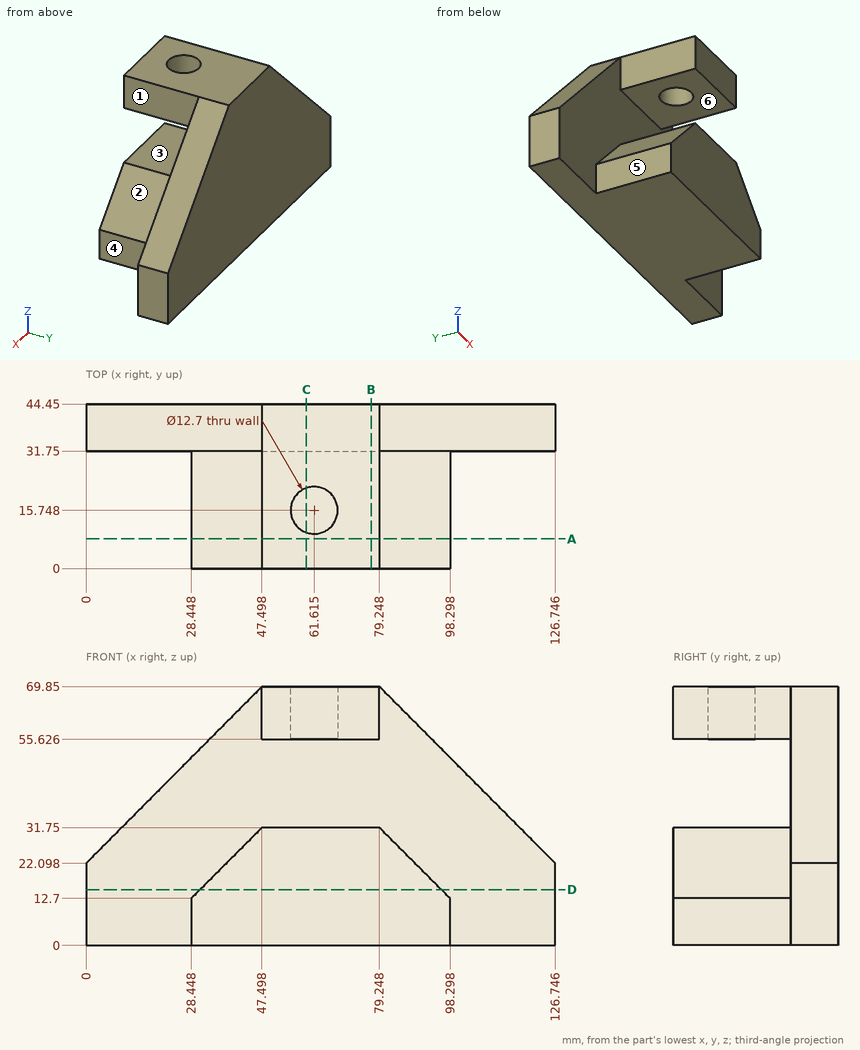
Input: dimensioned drawing with shaded views. Units: mm. Origin: part minimum x, y, z. A direction names the side the tool comes from. Coordinates: 2 decimals unless noted, no trailing zeros. Loops run counter-clockwise (first coordinate to the right, second up) from the corner with the lowest first, then second, coordinate; pieces in that order, holes last. Notation, with made-up numbers: M 32.25,28.5 L 56.25,28.5 A16 ccw 56.25,37.5 Z; hole C 12.25,-22 d4. An arc over 180 degrees is marked long. Use a Markdown table: item, result. Add a question column.
1) Section D-D, the plane z = 15. Return the cut outline in (x, y).
2) Draft query along Z for the marked faces 1, 2 and 3. Return one class per face: +Z half, -Z half, draft (parallel to the pull), parting line (faces both ways), or undercut.
3) Section B-B, the plane x = 77. Return the cut outline in (y, z), plus the area to 3 significant figures.
4) Pin query (flat end, axial travel): P1, Ø12, axis at x = 100.5, y = 8.5, coming from the +Z side; P2, Ø6, axis at y = 15, z = 59, coming from the -X side; P3, Ø7, axis at y = 12.5, z = 62.5, coming from the +X side; P4, Ø1.5, axis at x = 100, y = 5, coming from the -Z side. Return the tip coordinate at first contact, or that it passes through.
5) Line query: L1, parallel to Z at x = 64, y = 31.5; L2, parallel to Y at x = 41, z = 55; L3, parallel to X at y = 29, z = 59.5. Output: solid intervals per line, ascending. Write a range as from..to.
6) Section C-C, the plane x = 59.5. Return the cut outline in (y, z), plus the area to 3 significant figures.
7) Set-up query: the marked faces 4, 5 and 6. Return all of +Z, -Z, +X, -X, +Y, -Y with unobstructed straight access to the full face (end or side cutting, diameter ignored); none if empty.
8) Section A-A, the plane y = 8. Return the cut outline in (x, z).
Answer below:
| question | item | result |
|---|---|---|
| 1 | outline | M 0,31.75 L 30.75,31.75 L 30.75,0 L 96,0 L 96,31.75 L 126.75,31.75 L 126.75,44.45 L 0,44.45 Z |
| 2 | face 1 | draft |
| 2 | face 2 | +Z half |
| 2 | face 3 | undercut |
| 3 | outline | M 0,0 L 44.45,0 L 44.45,69.85 L 0,69.85 L 0,55.63 L 31.75,55.63 L 31.75,31.75 L 0,31.75 Z |
| 3 | area | 2,350 mm2 |
| 4 | P1 | z = 16.5 |
| 4 | P2 | x = 47.5 |
| 4 | P3 | x = 79.25 |
| 4 | P4 | through |
| 5 | L1 | 0..31.75, 55.63..69.85 |
| 5 | L2 | 31.75..44.45 |
| 5 | L3 | 47.5..79.25 |
| 6 | outline | M 0,0 L 44.45,0 L 44.45,69.85 L 21.74,69.85 L 21.74,55.63 L 31.75,55.63 L 31.75,31.75 L 0,31.75 Z; M 0,55.63 L 9.76,55.63 L 9.76,69.85 L 0,69.85 Z |
| 6 | area | 2,180 mm2 |
| 7 | face 4 | +Z, -Z, +X, -Y |
| 7 | face 5 | +Z, -Z, -X, -Y |
| 7 | face 6 | +X, -X, -Y |
| 8 | outline | M 28.45,0 L 98.3,0 L 98.3,12.7 L 79.25,31.75 L 47.5,31.75 L 28.45,12.7 Z; M 47.5,55.63 L 79.25,55.63 L 79.25,69.85 L 47.5,69.85 Z |
